Design review of the part built by this model. Coordinates are the model's own, in mm. A direction names the side the tool comes from. Round coordinates to 2 decimals unless told otherwise and drop trailing zeros. Write each loop counter-clockwise with the first axis right and the second up, starting at its lowest first coordinate (ties: lowest second). Pieces come first, ordered by that corner, then holes. Notation, with made-up numbers: (54.25, -33) - (70.25, -33) arc R18 cw to (70.25, -28) - close; hole circle Ø10 at (-8, 9). An arc over 180 degrees is marked (long way). Use one line per item in the form item = value.
```python
from build123d import *

# Parameters (mm, degrees)
SKETCH_1_W          = 20
SKETCH_1_H          = 29
SKETCH_1_R          = 1.5
EXTRUDE_1_DEPTH     = 4
SKETCH_2_W          = 20
SKETCH_2_H          = 4
EXTRUDE_2_DEPTH     = 18
CUT_EXTRUDE_1_DEPTH = 38.749172176
FILLET_1_R          = 10


with BuildPart() as part:
    # 草图1 → 凸台-拉伸1 (new body)
    with BuildSketch(Plane.XY):
        Rectangle(SKETCH_1_W, SKETCH_1_H)
        with Locations((5, 7.5)):
            Circle(SKETCH_1_R, mode=Mode.SUBTRACT)
        with Locations((-5, 7.5)):
            Circle(SKETCH_1_R, mode=Mode.SUBTRACT)
        with Locations((-5, -7.5)):
            Circle(SKETCH_1_R, mode=Mode.SUBTRACT)
        with Locations((5, -7.5)):
            Circle(SKETCH_1_R, mode=Mode.SUBTRACT)
    extrude(amount=EXTRUDE_1_DEPTH)

    # 草图2 → 凸台-拉伸2 (add)
    with BuildSketch(Plane.XY.offset(4)):
        with Locations((0, 12.5)):
            Rectangle(SKETCH_2_W, SKETCH_2_H)
        with Locations((0, -12.5)):
            Rectangle(SKETCH_2_W, SKETCH_2_H)
    extrude(amount=EXTRUDE_2_DEPTH)

    # 草图3 → 切除-拉伸1 (cut, through all)
    with BuildSketch(Plane.XZ.offset(14.5)):
        with BuildLine():
            ThreePointArc((2.5, 14.5), (0, 17), (-2.5, 14.5))
            Line((-2.5, 14.5), (2.5, 14.5))
        make_face()
        with BuildLine():
            Line((2.5, 14.5), (-2.5, 14.5))
            ThreePointArc((-2.5, 14.5), (0, 12), (2.5, 14.5))
        make_face()
    extrude(amount=-CUT_EXTRUDE_1_DEPTH, mode=Mode.SUBTRACT)

    # 圆角1
    fillet_1_edges = [part.edges().sort_by_distance(p)[0] for p in [
        (10, -12.5, 22),
        (10, 12.5, 22),
        (-10, 12.5, 22),
        (-10, -12.5, 22),
    ]]
    fillet(fillet_1_edges, radius=FILLET_1_R - 0.0001)  # a hair under: the kernel refuses the full size


solid = part.part
```
Q1. For P1, Ø4.5, axis at x = 0, z = 14.5, coming from the -Y side; P2, Ø6, axis at x = 7, y = -8, coming from the +Z side; P3, Ø4, axis at x = -5, y = 7.5, coming from the +Z side, all flat-tipped, find the tip position at first contact; note any pin that passes through.
Calculated:
P1 = through
P2 = 20.45
P3 = 4
Q2. To check wall thickness, follow line 1 along Y through (x, z) = (-5, 2.7); line 2 along Y through (x, z) = (-8, 5.75); line 3 along Z through (x, y) = (0, 12.05). State the ranges of each line that lie inside material, in increasing order. Write a range as from..to.
Calculated:
line_1 = -14.5..-9, -6..6, 9..14.5
line_2 = -14.5..-10.5, 10.5..14.5
line_3 = 0..12, 17..22
Q3. We need section B-B on z = 1.5. Write out the cut boundary in (x, y), then the cut area to 3 significant figures.
Calculated:
outline = (-10, -14.5) - (10, -14.5) - (10, 14.5) - (-10, 14.5) - close; hole circle Ø3 at (-5, -7.5); hole circle Ø3 at (-5, 7.5); hole circle Ø3 at (5, -7.5); hole circle Ø3 at (5, 7.5)
area = 552 mm2
Q4. We need section D-D on y = -2.75. Write out the cut boundary in (x, z), then the cut area to 3 significant figures.
Calculated:
outline = (-10, 0) - (10, 0) - (10, 4) - (-10, 4) - close
area = 80.0 mm2
Q5. We need section C-C on x = 5. Write out the cut boundary in (y, z).
Calculated:
outline = (-14.5, 0) - (-9, 0) - (-9, 4) - (-10.5, 4) - (-10.5, 20.66) - (-14.5, 20.66) - close; (-6, 0) - (6, 0) - (6, 4) - (-6, 4) - close; (9, 0) - (14.5, 0) - (14.5, 20.66) - (10.5, 20.66) - (10.5, 4) - (9, 4) - close
Q6. We need section A-A on z = 7. Write out the cut boundary in (x, y).
Calculated:
outline = (-10, -14.5) - (10, -14.5) - (10, -10.5) - (-10, -10.5) - close; (-10, 10.5) - (10, 10.5) - (10, 14.5) - (-10, 14.5) - close
Q7. Draft analysis for pull direction Z (two halves, no side actions). For faces 1 (the cylindrical face through (-7.15, -12.47, 18.99)), 2 (the cylindrical face through (0.54, 12.47, 16.94)), 3 (the flat face through (0, -10.5, 11)), state which applies: released by +Z, released by -Z, zero draft, split by the parting line, or undercut.
Calculated:
face_1 = released by +Z
face_2 = undercut
face_3 = zero draft
Q8. Machinability: for faces 4 (the cylindrical face through (-5, 6, 2)), 5 (the flat face through (0, 10.5, 11)), which of the approach directions +Z, -Z, +X, -X, +Y, -Y give a long, thin tool a straight path to every point of the face, cutting with its end or side? Answer none if there is none.
Calculated:
face_4 = +Z, -Z
face_5 = +Z, +X, -X
